```python
from build123d import *

# Parameters (mm, degrees)
BOSS_EXTRUDE1_DEPTH = 108.9
SKETCH2_R           = 19.075
BOSS_EXTRUDE2_DEPTH = 76
BOSS_EXTRUDE3_DEPTH = 22.9
SKETCH4_W           = 17.5
SKETCH4_H           = 17.5
BOSS_EXTRUDE4_DEPTH = 18
SKETCH5_R           = 3.25
CUT_EXTRUDE1_DEPTH  = 17.5
SKETCH6_R           = 10
CUT_EXTRUDE2_DEPTH  = 79


with BuildPart() as part:
    # Sketch1 → Boss-Extrude1 (new body)
    with BuildSketch(Plane(origin=(0, 0, 0), x_dir=(1, 0, 0), z_dir=(0, 1, 0))):
        with BuildLine():
            ThreePointArc((10.190041387, 10.664218515), (3.028324854, 14.435780151), (-5.045314834, 13.860277711))
            ThreePointArc((-5.045314834, 13.860277711), (-9.413082328, 16.626544393), (-11.770381199, 12.025156963))
            Line((-11.770381199, 12.025156963), (-19.909262437, 9.75))
            Line((-19.909262437, 9.75), (-19.909262437, -9.75))
            Line((-19.909262437, -9.75), (-11.770381199, -12.025156963))
            ThreePointArc((-11.770381199, -12.025156963), (-9.413082328, -16.626544393), (-5.045314834, -13.860277711))
            ThreePointArc((-5.045314834, -13.860277711), (3.028324854, -14.435780151), (10.190041387, -10.664218515))
            ThreePointArc((10.190041387, -10.664218515), (16.352409168, -11.515151515), (13.474496198, -6.000037683))
            ThreePointArc((13.474496198, -6.000037683), (14.75, 0), (13.474496198, 6.000037683))
            ThreePointArc((13.474496198, 6.000037683), (16.352409168, 11.515151515), (10.190041387, 10.664218515))
        make_face()
    extrude(amount=BOSS_EXTRUDE1_DEPTH)



with BuildPart() as body_2:
    # Sketch2 → Boss-Extrude2 (new body)
    with BuildSketch(Plane(origin=(0, 0, 0), x_dir=(1, 0, 0), z_dir=(0, 1, 0))):
        with Locations(Location((36.015737563, 0, 0), (0, 0, 270))):
            Circle(SKETCH2_R)
    extrude(amount=BOSS_EXTRUDE2_DEPTH)


with BuildPart() as part_1:
    add(part.part)

    add(body_2.part)  # Boss-Extrude3 merges body 2
    # Sketch3 → Boss-Extrude3 (add)
    with BuildSketch(Plane(origin=(0, 0, 0), x_dir=(1, 0, 0), z_dir=(0, 1, 0))):
        with BuildLine():
            Line((-19.909262437, 20.25), (-19.909262437, -20.25))
            Line((-19.909262437, -20.25), (35.440737563, -20.25))
            ThreePointArc((35.440737563, -20.25), (55.690737563, 0), (35.440737563, 20.25))
            Line((35.440737563, 20.25), (-19.909262437, 20.25))
        make_face()
    extrude(amount=-BOSS_EXTRUDE3_DEPTH)

    # Sketch4 → Boss-Extrude4 (add)
    with BuildSketch(Plane.XZ.offset(22.9)):
        with Locations((0.240737563, 0)):
            Rectangle(SKETCH4_W, SKETCH4_H)
    extrude(amount=BOSS_EXTRUDE4_DEPTH)

    # Sketch5 → Cut-Extrude1 (cut)
    with BuildSketch(Plane(origin=(0, 0, -8.75), x_dir=(-1, 0, 0), z_dir=(0, 0, -1))):
        with Locations((-0.240737563, -32.95)):
            Circle(SKETCH5_R)
    extrude(amount=-CUT_EXTRUDE1_DEPTH, mode=Mode.SUBTRACT)

    # Sketch6 → Cut-Extrude2 (cut)
    with BuildSketch(Plane(origin=(0, 108.9, 0), x_dir=(1, 0, 0), z_dir=(0, 1, 0))):
        with Locations(Location((0, 0, 0), (0, 0, 270))):
            Circle(SKETCH6_R)
    extrude(amount=-CUT_EXTRUDE2_DEPTH, mode=Mode.SUBTRACT)


solid = part_1.part
```
Geometry: final body of the model. Coordinates: model frame, mm. A direction names the side the tool comes from. Coordinates: 2 decimals unless noted, no trailing zeros. Order: outer loops, then holes, each group sorted by start corner. A loop starts at its lowest first (then second) coordinate and runs counter-clockwise, first axis right, second up. Notation, with made-up numbers: (45.25, 37.5) - (100.25, 37.5) arc R17 cw to (100.25, 49.5) - close; hole circle Ø6 at (79.5, 8). An arc over 180 degrees is marked (long way). Return JSON: item names as keys, results as strings. Group by question number.
1. Set-up query: faces 1 (the face through (0.664, -29.728, -0.123)), 2 (the face through (8.991, -32, 0)), 3 (the face through (-9.76, 69.95, -2.17)), 4 (the face through (2, -30, 8.75)), 5 (the face through (36, 76, 0)). Return all of +Z, -Z, +X, -X, +Y, -Y with unobstructed straight access to the full face (end or side cutting, diameter ignored); none if empty.
2. Cut plane A-A (y = -32.95). Output: boundary loops of the cut face in (x, z), plus the area to 4 significant figures.
3. Material intervals for line 1 along X through (y, z) = (48, 0); line 2 along X through (y, z) = (31.5, 8); line 3 along Y through (x, z) = (8.5, 12.5), sorted ascending. Write a range as [from, to].
4. Pin query (flat end, axial travel): pin 1 (5 mm diameter, centred on y = -35.5, z = 3, fed in from -X); pin 2 (8 mm diameter, centred on x = 19, z = 0, fed in from +Y); pin 3 (10.5 mm diameter, centred on x = 0.24, y = -32.95, fed in from +Z). Return the tip coordinate at first contact, or that it passes through.
5. Cut plane D-D (x = 0). Output: boundary loops of the cut face in (y, z), plus the area to 3 significant figures.
6. Pull-direction query (Z, two-part tool) for faces 6 (the face through (14.75, 53.69, 0.09)), 7 (the face through (-8.509, -32, 0)), 8 (the face through (8, -11, -20.25)); classes: pulls with the +Z half, pulls with the -Z half, needs draft (parallel to the pull), parting line crosses it, or undercut.
7. Cut plane B-B (z = 0). Output: boundary loops of the cut face in (x, y), plus the area to 3 significant figures.
8. Cut plane C-C (y = 59). Count the separate pieces of the cut face and the enclosed holes in it, plus the area to 3 significant figures.
Resolved:
{
 "1": {"face 1": "+Z, -Z", "face 2": "+Z, -Z, +X, -Y", "face 3": "+Y", "face 4": "+Z, +X, -X, -Y", "face 5": "+Z, -Z, +X, +Y"},
 "2": {"outline": "(-8.51, -8.75) - (-3.01, -8.75) - (-3.01, 8.75) - (-8.51, 8.75) - close; (3.49, -8.75) - (8.99, -8.75) - (8.99, 8.75) - (3.49, 8.75) - close", "area": "192.5 mm²"},
 "3": {"line 1": "x = [-19.91, -10], [10, 14.75], [16.94, 55.09]", "line 2": "x = [-19.91, -6], [6, 16.65], [18.7, 53.33]", "line 3": "y = [-22.9, 0]"},
 "4": {"pin 1": "stops at x = -8.51", "pin 2": "stops at y = 76", "pin 3": "stops at z = 8.75"},
 "5": {"outline": "(-40.9, -8.75) - (-36.19, -8.75) - (-36.19, 8.75) - (-40.9, 8.75) - close; (-29.71, -8.75) - (-22.9, -8.75) - (-22.9, -20.25) - (0, -20.25) - (0, -14.75) - (108.9, -14.75) - (108.9, -10) - (29.9, -10) - (29.9, 10) - (108.9, 10) - (108.9, 14.75) - (0, 14.75) - (0, 20.25) - (-22.9, 20.25) - (-22.9, 8.75) - (-29.71, 8.75) - close", "area": "2,760 mm²"},
 "6": {"face 6": "undercut", "face 7": "needs draft", "face 8": "pulls with the -Z half"},
 "7": {"outline": "(-19.91, -22.9) - (-8.51, -22.9) - (-8.51, -40.9) - (8.99, -40.9) - (8.99, -22.9) - (55.69, -22.9) - (55.69, 0) - (55.09, 0) - (55.09, 76) - (16.94, 76) - (16.94, 0) - (14.75, 0) - (14.75, 108.9) - (10, 108.9) - (10, 29.9) - (-10, 29.9) - (-10, 108.9) - (-19.91, 108.9) - close; hole circle Ø6.5 at (0.24, -32.95)", "area": "7,110 mm²"},
 "8": {"separate pieces": "2", "enclosed holes": "1", "area": "1,770 mm²"}
}
